Build history of the part. All positions in model axes, mm. Give positions to 0.01 mm unless a question says otherwise; leave off trailing zeros. Write each loop counter-clockwise with the first axis right and the second up, starting at its lowest first coordinate (ties: lowest second). Pieces come first, ordered by that corner, then holes. Notation, with made-up numbers: M 24.25,73.5 L 68.25,73.5 A30 ccw 68.25,110.5 Z; hole C -27,-3 d3. An arc over 180 degrees is marked long. Return JSON: item names as keys, results as strings. Group by question number.
Q1. Band-saw the part on B-B, the plane y = 23.5. Give the cut face in (x, z) (3 decimals), then the cut area to 3 significant figures.
Q2. Wall check: probe 1 along X at (y, z) = (-9, 1.4) (3 decimals); probe 2 along Y at (x, z) = (57, 1); probe 3 along Y at (x, z) = (-39, 0.35). Give the ranges that are in metal, low to high.
Q3. Band-saw the part on D-D, the plane x = 62. Give the cut face in (y, z).
Q4. Flat gauge pins, fed straight in: pin 1 Ø3.5 at (x, y) = (-36.28, -5.36) entering from +Z; pin 2 Ø1 at (x, z) = (15.5, 0.5) entering from +Y. Where does each tip first touch, or does it go through?
Q5. Band-saw the part on A-A, the plane x = -59. Give the cut face in (y, z), then the cut area to 3 significant figures.
Q6. Band-saw the part on C-C, the plane y = -14.5. Count the separate pieces of the cut face and the enclosed holes in it, then the cut area to 3 significant figures.
from build123d import *

# Parameters (mm, degrees)
SKETCH_1_W             = 158.45
SKETCH_1_H             = 60
EXTRUDE_1_DEPTH        = 2
SKETCH_2_R             = 1.6
CUT_EXTRUDE_1_DEPTH    = 10
EXTRUDE_2_DEPTH        = 2
CUT_EXTRUDE_2_DEPTH    = 10
PATTERN_LINEAR_1_COUNT = 6
PATTERN_LINEAR_1_PITCH = 24.9
FILLET_1_R             = 5
CUT_EXTRUDE_3_DEPTH    = 10
SKETCH_6_W             = 15
SKETCH_6_H             = 21.8
EXTRUDE_3_DEPTH        = 2
SKETCH_7_R             = 2.05
CUT_EXTRUDE_4_DEPTH    = 10
FILLET_2_R             = 2
SKETCH_8_W             = 18
SKETCH_8_H             = 2
CUT_EXTRUDE_5_DEPTH    = 1
FILLET_3_R             = 0.5


with BuildPart() as part:
    # 草图1 → 凸台-拉伸1 (new body)
    with BuildSketch(Plane.XY):
        Rectangle(SKETCH_1_W, SKETCH_1_H)
    extrude(amount=EXTRUDE_1_DEPTH)

    # 草图2 → 切除-拉伸1 (cut)
    with BuildSketch(Plane.XY.offset(2)):
        with Locations((-76.225, -14.5)):
            Circle(SKETCH_2_R)
        with Locations((-76.225, 5.5)):
            Circle(SKETCH_2_R)
        with Locations((76.225, -14.5)):
            Circle(SKETCH_2_R)
        with Locations((76.225, 5.5)):
            Circle(SKETCH_2_R)
    extrude(amount=-CUT_EXTRUDE_1_DEPTH, mode=Mode.SUBTRACT)

    # 草图3 → 凸台-拉伸2 (add)
    with BuildSketch(Plane(origin=(0, 0, 0), x_dir=(-1, 0, 0), z_dir=(0, 0, -1))):
        Polygon((-79.225, 30), (-79.225, 50), (79.225, 37), (79.225, 30), align=None)
    extrude(amount=-EXTRUDE_2_DEPTH)

    # 草图4 → 切除-拉伸2 (cut)
    with BuildSketch(Plane(origin=(0, 0, 0), x_dir=(-1, 0, 0), z_dir=(0, 0, -1))):
        with BuildLine():
            Line((-56.225, 21.5), (-56.225, -17.5))
            ThreePointArc((-56.225, -17.5), (-63.725, -25), (-71.225, -17.5))
            Line((-71.225, -17.5), (-71.225, 21.5))
            ThreePointArc((-71.225, 21.5), (-63.725, 29), (-56.225, 21.5))
        make_face()
    cut_extrude_2 = extrude(amount=-CUT_EXTRUDE_2_DEPTH, mode=Mode.SUBTRACT)

    # 阵列(线性)1: 切除-拉伸2 ×6
    with Locations(*[(-i * PATTERN_LINEAR_1_PITCH, 0, 0) for i in range(1, PATTERN_LINEAR_1_COUNT)]):
        add(cut_extrude_2, mode=Mode.SUBTRACT)

    # 圆角1
    fillet_1_edges = [part.edges().sort_by_distance(p)[0] for p in [
        (79.225, 50, 1),
        (-79.225, 37, 1),
        (79.225, -30, 1),
        (-79.225, -30, 1),
    ]]
    fillet(fillet_1_edges, radius=FILLET_1_R)

    # 草图5 → 切除-拉伸3 (cut)
    with BuildSketch(Plane(origin=(0, 0, 0), x_dir=(-1, 0, 0), z_dir=(0, 0, -1))):
        with BuildLine():
            Line((-69.607368079, 45.699163119), (-19.774807001, 41.610660159))
            ThreePointArc((-19.774807001, 41.610660159), (-18.402485258, 39.993028237), (-20.020117179, 38.620706494))
            Line((-20.020117179, 38.620706494), (-69.852678256, 42.709209454))
            ThreePointArc((-69.852678256, 42.709209454), (-71.225, 44.326841375), (-69.607368079, 45.699163119))
        make_face()
        with BuildLine():
            Line((14.515094011, 38.797351776), (64.347655089, 34.708848816))
            ThreePointArc((64.347655089, 34.708848816), (65.719976832, 33.091216895), (64.102344911, 31.718895152))
            Line((64.102344911, 31.718895152), (14.269783834, 35.807398112))
            ThreePointArc((14.269783834, 35.807398112), (12.89746209, 37.425030033), (14.515094011, 38.797351776))
        make_face()
    extrude(amount=-CUT_EXTRUDE_3_DEPTH, mode=Mode.SUBTRACT)

    # 草图6 → 凸台-拉伸3 (add)
    with BuildSketch(Plane.XY.offset(2)):
        with Locations((-35.875, 0.6)):
            Rectangle(SKETCH_6_W, SKETCH_6_H)
    extrude(amount=-EXTRUDE_3_DEPTH)

    # 草图7 → 切除-拉伸4 (cut)
    with BuildSketch(Plane.XY.offset(2)):
        with Locations((-37.261557274, 6.6)):
            Circle(SKETCH_7_R)
        with Locations((-36.280316563, -5.359814659)):
            Circle(SKETCH_7_R)
    extrude(amount=-CUT_EXTRUDE_4_DEPTH, mode=Mode.SUBTRACT)

    # 圆角2
    fillet_2_edges = [part.edges().sort_by_distance(p)[0] for p in [
        (-28.375, -10.3, 1),
        (-28.375, 11.5, 1),
        (-43.375, 11.5, 1),
        (-43.375, -10.3, 1),
    ]]
    fillet(fillet_2_edges, radius=FILLET_2_R)

    # 草图8 → 切除-拉伸5 (cut)
    with BuildSketch(Plane(origin=(-3.545085978, 43.209144098, 0), x_dir=(0.9966512215507048, 0.08177005919948983, 0), z_dir=(-0.08177005919948983, 0.9966512215507048, 0))):
        with Locations((-38.57643531, -1)):
            Rectangle(SKETCH_8_W, SKETCH_8_H)
    extrude(amount=-CUT_EXTRUDE_5_DEPTH, mode=Mode.SUBTRACT)

    # 圆角3
    fillet_3_edges = [part.edges().sort_by_distance(p)[0] for p in [
        (-50.880428288, 38.322164944, 1),
        (-32.9407063, 39.79402601, 1),
    ]]
    fillet(fillet_3_edges, radius=FILLET_3_R)
    fillet_3_2_edges = [part.edges().sort_by_distance(p)[0] for p in [
        (-50.962198347, 39.318816166, 1),
        (-33.022476359, 40.790677231, 1),
    ]]
    fillet(fillet_3_2_edges, radius=FILLET_3_R - 0.0001)  # a hair under: the kernel refuses the full size


solid = part.part
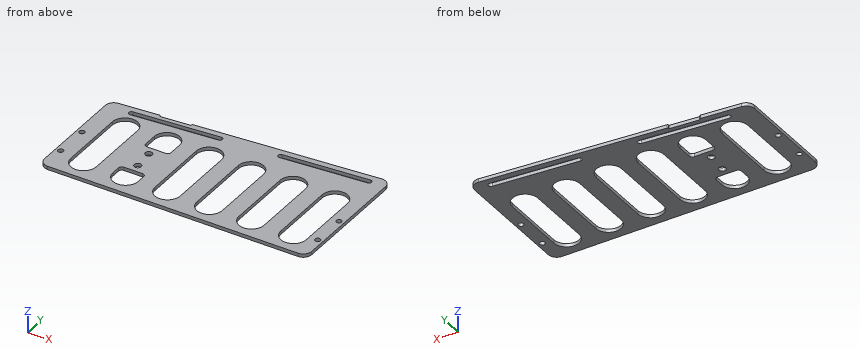
From the geometry:
{
 "1": {"outline": "M -79.225,0 L -68.003,0 L -68.003,2 L -79.225,2 Z; M -53.547,0 L -43.103,0 L -43.103,2 L -53.547,2 Z; M -28.647,0 L -18.203,0 L -18.203,2 L -28.647,2 Z; M -3.747,0 L 6.697,0 L 6.697,2 L -3.747,2 Z; M 21.153,0 L 31.597,0 L 31.597,2 L 21.153,2 Z; M 46.053,0 L 56.497,0 L 56.497,2 L 46.053,2 Z; M 70.953,0 L 79.225,0 L 79.225,2 L 70.953,2 Z", "area": "143 mm^2"},
 "2": {"probe 1": "x = -79.225 to -68.275, -53.275 to -18.475, -3.475 to 6.425, 21.425 to 31.325, 46.325 to 56.225, 71.225 to 79.225", "probe 2": "y = -30 to -20.82, 24.82 to 41.65, 44.66 to 48.18", "probe 3": "y = -30 to -24.32, -10.3 to 5.51, 7.69 to 11.5, 28.32 to 33.78, 36.79 to 39.3"},
 "3": {"outline": "M -30,0 L -24.8,0 L -24.8,2 L -30,2 Z; M 28.8,0 L 42.06,0 L 42.06,2 L 28.8,2 Z; M 45.08,0 L 48.59,0 L 48.59,2 L 45.08,2 Z"},
 "4": {"pin 1": "passes through", "pin 2": "stops at y = 44.81"},
 "5": {"outline": "M -30,0 L -24.79,0 L -24.79,2 L -30,2 Z; M 28.79,0 L 32.14,0 L 32.14,2 L 28.79,2 Z; M 35.15,0 L 38.66,0 L 38.66,2 L 35.15,2 Z", "area": "24.2 mm^2"},
 "6": {"separate pieces": "9", "enclosed holes": "0", "area": "124 mm^2"}
}
